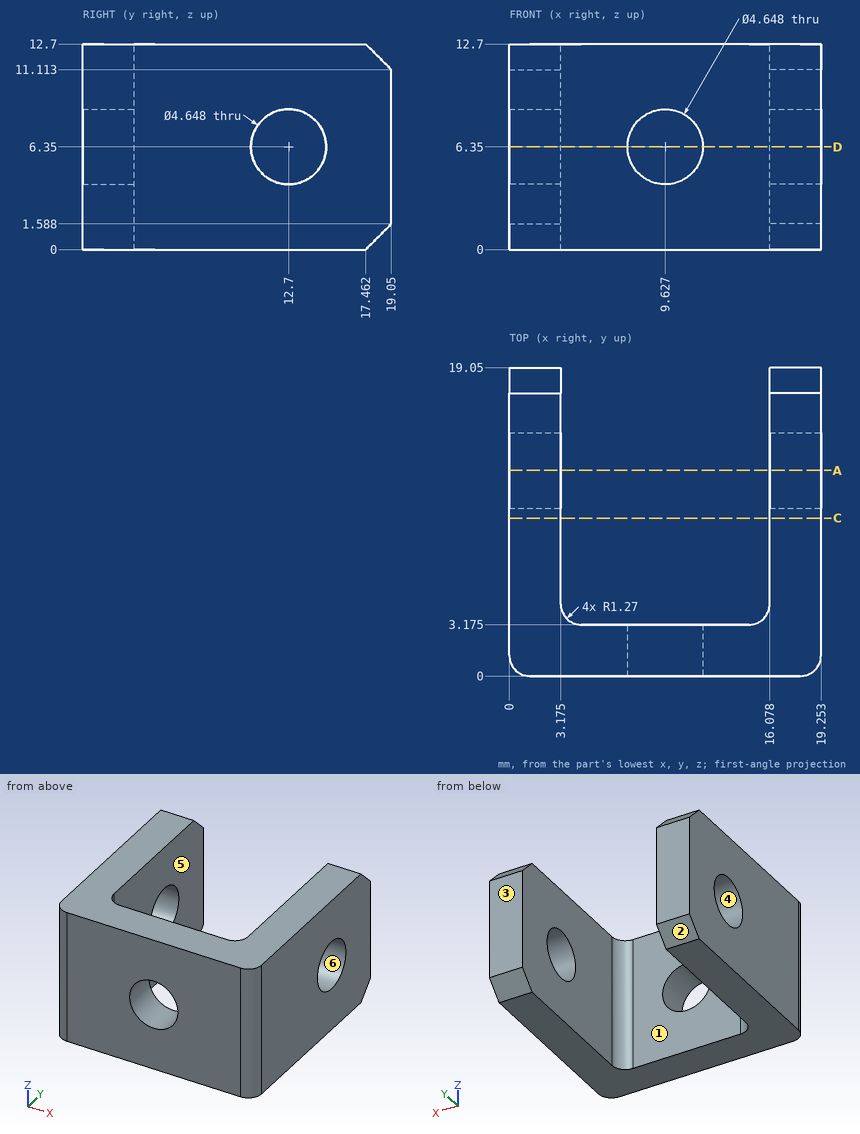
Could you check a few things on this drawing? It's one solid part, dimensions in mm from its lowest x, y, z. A direction names the side the tool comes from. Coordinates: 2 decimals unless noted, no trailing zeros. Order: outer loops, then holes, each group sorted by start corner. A loop starts at its lowest first (then second) coordinate and runs counter-clockwise, first axis right, second up. Notation, with made-up numbers: (38.5, -1.75) - (66.5, -1.75) arc R29 ccw to (66.5, 37.25) - close; hole circle Ø1 at (68.5, 66.5). An arc over 180 degrees is marked (long way). Answer as a JSON object with one key per item and string values. Group by question number.
Q1. We'd pull the mould along Y, two halves only. Please class the marked faces 3, 4, 5 and 6: +Y half, -Y half, draft (parallel to the pull), parting line (faces both ways), or undercut.
Q2. Imagine slicing it at A-A (y = 12.7). Please give me the cut outline in (x, z) (1 decimal).
Q3. I need wall thicknesses on line 1 (X direction, y = 4.5, z = 3.5) (1 decimal); line 2 (Y direction, x = 5.25, z = 9.5) (1 decimal); line 3 (X direction, y = 1.7, z = 6.35). Which ranges of each line are inside material? Lowest first, please. Write a range as from..to.
Q4. On a 3-axis mill with a long thin cutter (end or side, diameter ignored), from which of +Z, -Z, +X, -X, +Y, -Y can I reach the whole of each face in a straight line? I mean the marked faces 1 and 2. Say none if no direction works.
Q5. Imagine slicing it at C-C (y = 9.75). Please give me the cut outline in (x, z) (1 decimal).
Q6. Imagine slicing it at D-D (z = 6.35). Give the number of separate pieces and of enclosed holes in the cut face, and give its area (3 significant figures).
Determined:
{
 "1": {"face 3": "+Y half", "face 4": "undercut", "face 5": "draft", "face 6": "undercut"},
 "2": {"outline": "(0, 0) - (3.2, 0) - (3.2, 4) - (0, 4) - close; (0, 8.7) - (3.2, 8.7) - (3.2, 12.7) - (0, 12.7) - close; (16.1, 0) - (19.3, 0) - (19.3, 4) - (16.1, 4) - close; (16.1, 8.7) - (19.3, 8.7) - (19.3, 12.7) - (16.1, 12.7) - close"},
 "3": {"line 1": "x = 0..3.2, 16.1..19.3", "line 2": "y = 0..3.2", "line 3": "x = 0..7.3, 11.95..19.25"},
 "4": {"face 1": "+Z, -Z, +Y", "face 2": "-Z, +X, -X, +Y"},
 "5": {"outline": "(0, 0) - (3.2, 0) - (3.2, 12.7) - (0, 12.7) - close; (16.1, 0) - (19.3, 0) - (19.3, 12.7) - (16.1, 12.7) - close"},
 "6": {"separate pieces": "4", "enclosed holes": "0", "area": "118 mm2"}
}
